Design review of the part built by this model. Coordinates are the model's own, in mm. Face numbers are marked on the shaded views. A direction names the side the tool comes from. Coordinates: 2 decimals unless noted, no trailing zeros. Loops run counter-clockwise (first coordinate to the right, second up) from the corner with the lowest first, then second, coordinate; pieces in that order, holes last. Notation, with made-up numbers: (-17, 40.5) - (35, 40.5) arc R13 cw to (35, 61.5) - close; hole circle Ø8 at (87.25, 21). An arc over 180 degrees is marked (long way). Return JSON: item names as keys, results as strings. Group by question number.
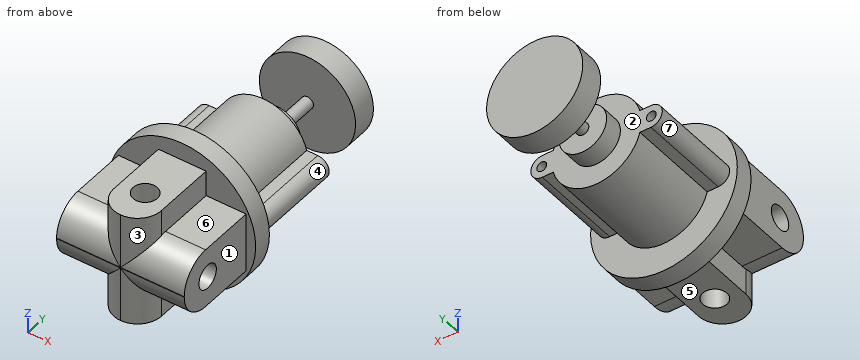
from build123d import *

# Parameters (mm, degrees)
BOSS_EXTRUDE1_DEPTH        = 49
F_1_4_20_TAPPED_HOLE1_D    = 5.1054
SKETCH4_R                  = 38.5
BOSS_EXTRUDE2_DEPTH        = 10
BOSS_EXTRUDE3_DEPTH        = 45
FILLET1_R                  = 12.5
FILLET2_R                  = 15.5
F_1_2_0_5_DIAMETER_HOLE1_D = 12.7
F_1_2_0_5_DIAMETER_HOLE2_D = 12.7
SKETCH10_R                 = 12.5
BOSS_EXTRUDE4_DEPTH        = 10
SKETCH11_R                 = 3.175
BOSS_EXTRUDE5_DEPTH        = 22
SKETCH12_R                 = 25.25
BOSS_EXTRUDE6_DEPTH        = 13


with BuildPart() as part:
    # Sketch1 → Boss-Extrude1 (new body)
    with BuildSketch(Plane(origin=(0, 0, 0), x_dir=(1, 0, 0), z_dir=(0, 1, 0))):
        with BuildLine():
            Line((-28.5, 6), (-22.721135535, 6))
            ThreePointArc((-22.721135535, 6), (0, 23.5), (22.721135535, 6))
            Line((22.721135535, 6), (28.5, 6))
            ThreePointArc((28.5, 6), (34.5, 0), (28.5, -6))
            Line((28.5, -6), (22.721135535, -6))
            ThreePointArc((22.721135535, -6), (0, -23.5), (-22.721135535, -6))
            Line((-22.721135535, -6), (-28.5, -6))
            ThreePointArc((-28.5, -6), (-34.5, 0), (-28.5, 6))
        make_face()
    extrude(amount=-BOSS_EXTRUDE1_DEPTH)

    # 1/4-20 Tapped Hole1 (through all)
    with Locations(Plane(origin=(0, 0, 0), x_dir=(1, 0, 0), z_dir=(0, 1, 0))):
        with Locations((-28.75, 0), (28.75, 0)):
            Hole(F_1_4_20_TAPPED_HOLE1_D / 2)

    # Sketch4 → Boss-Extrude2 (add)
    with BuildSketch(Plane.XZ.offset(49)):
        with Locations(Location((0, 0, 0), (0, 0, 270))):
            Circle(SKETCH4_R)
    extrude(amount=BOSS_EXTRUDE2_DEPTH)

    # Sketch5 → Boss-Extrude3 (add)
    with BuildSketch(Plane.XZ.offset(59)):
        Polygon((12.5, 15.65), (33.5, 15.65), (33.5, -15.65), (12.5, -15.65), (12.5, -29.165), (-12.5, -29.165), (-12.5, -15.65), (-33.5, -15.65), (-33.5, 15.65), (-12.5, 15.65), (-12.5, 29.165), (12.5, 29.165), align=None)
    extrude(amount=BOSS_EXTRUDE3_DEPTH)

    # Fillet1
    fillet1_edges = [part.edges().sort_by_distance(p)[0] for p in [
        (12.5, -104, 22.4075),
        (-12.5, -104, 22.4075),
        (-12.5, -104, -22.4075),
        (12.5, -104, -22.4075),
    ]]
    fillet(fillet1_edges, radius=FILLET1_R - 0.0001)  # a hair under: the kernel refuses the full size

    # Fillet2
    fillet2_edges = [part.edges().sort_by_distance(p)[0] for p in [
        (-16.75005, -104, 15.65),
        (-16.75005, -104, -15.65),
        (16.75005, -104, 15.65),
        (16.75005, -104, -15.65),
    ]]
    fillet(fillet2_edges, radius=FILLET2_R)

    # 1/2 (0.5) Diameter Hole1 (through all)
    with Locations(Plane(origin=(0, 0, -29.165), x_dir=(-1, 0, 0), z_dir=(0, 0, -1))):
        with Locations((0, -86)):
            Hole(F_1_2_0_5_DIAMETER_HOLE1_D / 2)

    # 1/2 (0.5) Diameter Hole2 (through all)
    with Locations(Plane(origin=(33.5, 0, 0), x_dir=(0, 0, -1), z_dir=(1, 0, 0))):
        with Locations((0.125480769, -87)):
            Hole(F_1_2_0_5_DIAMETER_HOLE2_D / 2)

    # Sketch10 → Boss-Extrude4 (add)
    with BuildSketch(Plane(origin=(0, 0, 0), x_dir=(1, 0, 0), z_dir=(0, 1, 0))):
        with Locations(Location((0, 0, 0), (0, 0, 270))):
            Circle(SKETCH10_R)
    extrude(amount=BOSS_EXTRUDE4_DEPTH)

    # Sketch11 → Boss-Extrude5 (add)
    with BuildSketch(Plane(origin=(0, 10, 0), x_dir=(1, 0, 0), z_dir=(0, 1, 0))):
        with Locations(Location((0, 0, 0), (0, 0, 270))):
            Circle(SKETCH11_R)
    extrude(amount=BOSS_EXTRUDE5_DEPTH)

    # Sketch12 → Boss-Extrude6 (add)
    with BuildSketch(Plane(origin=(0, 32, 0), x_dir=(1, 0, 0), z_dir=(0, 1, 0))):
        with Locations(Location((0, 0, 0), (0, 0, 90))):
            Circle(SKETCH12_R)
    extrude(amount=BOSS_EXTRUDE6_DEPTH)


solid = part.part
Item 1: For the marked faces 4, 5, 6 and 7, list the 3-axis set-ups (+Z, -Z, +X, -X, +Y, -Y) from which the entire face can be reached by the end or side of a thin tool; tool diameter is ignored.
Item 2: Add section A-A (y = -12). State the section outline as (x, z) points.
Item 3: Add section B-B (y = -61). State the section outline as (x, z) points (3 decimals), then the cut area to 3 significant figures.
Item 4: To check wall thickness, follow line 1 (Z direction, x = -29.5, y = -87); line 2 (X direction, y = -86.5, z = 27); line 3 (X direction, y = -86, z = -10). State the ranges of each line that lie inside material, in increasing order. Write a range as from..to.
Item 5: Draft analysis for pull direction Y (two halves, no side actions). For the marked faces 1, 2 and 3, state which applies: pulls with the +Y half, pulls with the -Y half, needs draft (parallel to the pull), parting line crosses it, or undercut.
Item 6: For P1, Ø4.5, axis at x = -26, y = -29.5, coming from the +Z side; P2, Ø5, axis at x = 27.5, y = -83.5, coming from the +Z side; P3, Ø2.5, axis at x = 28, z = 1, coming from the +Y side, all flat-tipped, find the tip position at first contact; note any pin that passes through.
Answers below:
{
 "1": {"face 4": "+X, +Y", "face 5": "-Z, +X, -X, -Y", "face 6": "+Z, +X, -Y", "face 7": "-X, +Y"},
 "2": {"outline": "(-28.5, -6) - (-22.72, -6) arc R23.5 ccw to (22.72, -6) - (28.5, -6) arc R6 ccw to (28.5, 6) - (22.72, 6) arc R23.5 ccw to (-22.72, 6) - (-28.5, 6) arc R6 ccw to start; hole circle Ø5.11 at (-28.75, 0); hole circle Ø5.11 at (28.75, 0)"},
 "3": {"outline": "(-33.5, -15.65) - (-12.5, -15.65) - (-12.5, -29.165) - (12.5, -29.165) - (12.5, -15.65) - (33.5, -15.65) - (33.5, 15.65) - (12.5, 15.65) - (12.5, 29.165) - (-12.5, 29.165) - (-12.5, 15.65) - (-33.5, 15.65) - close", "area": "2,770 mm^2"},
 "4": {"line 1": "z = -15.65..-6.48, 6.22..15.65", "line 2": "x = -12.5..-6.33, 6.33..12.5", "line 3": "x = -33.5..-6.35, 6.35..33.5"},
 "5": {"face 1": "needs draft", "face 2": "undercut", "face 3": "pulls with the -Y half"},
 "6": {"P1": "stops at z = 6", "P2": "stops at z = 15.65", "P3": "stops at y = -49"}
}
